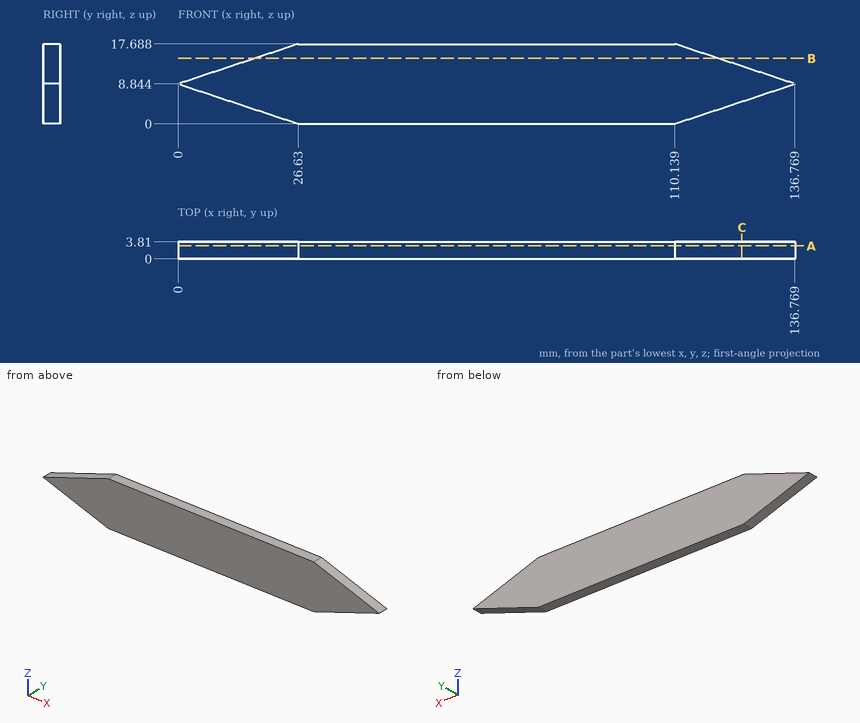
Verification items for this drawing (mm, ordinates from the low corner). Give positions to 0.01 mm unless a question says otherwise; leave off trailing zeros. Loops run counter-clockwise (first coordinate to the right, second up) from the corner with the lowest first, then second, coordinate; pieces in that order, holes last. Notation, with made-up numbers: M 14,64 L 42,64 A30 cw 42,89 Z; hole C -8,57.5 d5. An arc over 180 degrees is marked long. Return JSON: item names as keys, results as strings. Group by question number.
1. Cross-section at A-A on y = 2.9. Record the boundary of the cut face in (x, z), plus the area to 3 significant figures.
2. Cross-section at C-C on x = 125. Record the boundary of the cut face in (y, z) (1 decimal).
3. Cross-section at B-B on z = 14.5. Record the boundary of the cut face in (x, y), plus the area to 3 significant figures.
4. Thickness scan on L1, parallel to Z at x = 128, y = 2.95; L2, parallel to Z at x = 115.5, y = 1.25. Record the ranges inside material, lowest first.
Return value:
{
 "1": {"outline": "M 0,8.84 L 26.63,0 L 110.14,0 L 136.77,8.84 L 110.14,17.69 L 26.63,17.69 Z", "area": "1,950 mm^2"},
 "2": {"outline": "M 0,4.9 L 3.8,4.9 L 3.8,12.8 L 0,12.8 Z"},
 "3": {"outline": "M 17.03,0 L 119.74,0 L 119.74,3.81 L 17.03,3.81 Z", "area": "391 mm^2"},
 "4": {"L1": "5.93 to 11.76", "L2": "1.78 to 15.91"}
}
